Geometry: final body of the model. Coordinates: model frame, mm. Give positions to 0.01 mm unless a question says otherwise; leave off trailing zeros. Order: outer loops, then holes, each group sorted by start corner. A loop starts at its lowest first (then second) coordinate and runs counter-clockwise, first axis right, second up. Notation, with made-up numbers: (-29.5, 81.25) -> (12.5, 81.25) arc R29 cw to (12.5, 120.25) -> close; hole circle Ø11 at (86, 36.5). An arc over 180 degrees is marked (long way). One line per question, with ' | ' between items.
from build123d import *

# Parameters (mm, degrees)
ESQUISSE1_W             = 94.57
ESQUISSE1_H             = 60.88
BOSS_EXTRU_1_DEPTH      = 3.7
ESQUISSE2_W             = 88.629386258
ESQUISSE2_H             = 58.041323691
ENL_V_MAT_EXTRU_1_DEPTH = 0.05
ESQUISSE3_W             = 3.887425577
ESQUISSE3_H             = 19.495847756
BOSS_EXTRU_2_DEPTH      = 0.05
ESQUISSE4_W             = 3.887425577
ESQUISSE4_H             = 19.495847756
BOSS_EXTRU_3_DEPTH      = 0.1


with BuildPart() as part:
    # Esquisse1 → Boss.-Extru.1 (new body)
    with BuildSketch(Plane.XY):
        with Locations((47.285, 30.44)):
            Rectangle(ESQUISSE1_W, ESQUISSE1_H)
    extrude(amount=BOSS_EXTRU_1_DEPTH)

    # Esquisse2 → Enlèv. mat.-Extru.1 (cut)
    with BuildSketch(Plane.XY.offset(3.7)):
        with Locations((48.709909747, 30.392503009)):
            Rectangle(ESQUISSE2_W, ESQUISSE2_H)
    extrude(amount=-ENL_V_MAT_EXTRU_1_DEPTH, mode=Mode.SUBTRACT)

    # Esquisse3 → Boss.-Extru.2 (add)
    with BuildSketch(Plane(origin=(0, 0, 0), x_dir=(-1, 0, 0), z_dir=(0, 0, -1))):
        with BuildLine():
            Line((-9.099589702, 9.441066071), (0, 9.441066071))
            Line((0, 9.441066071), (0, 51.438933929))
            Line((0, 51.438933929), (-9.099589702, 51.438933929))
            ThreePointArc((-9.099589702, 51.438933929), (-10.513803264, 50.853147491), (-11.099589702, 49.438933929))
            Line((-11.099589702, 49.438933929), (-11.099589702, 42.94))
            ThreePointArc((-11.099589702, 42.94), (-11.68537614, 41.525786438), (-13.099589702, 40.94))
            Line((-13.099589702, 40.94), (-40, 40.94))
            Line((-40, 40.94), (-40, 19.94))
            Line((-40, 19.94), (-13.099589702, 19.94))
            ThreePointArc((-13.099589702, 19.94), (-11.68537614, 19.354213562), (-11.099589702, 17.94))
            Line((-11.099589702, 17.94), (-11.099589702, 11.441066071))
            ThreePointArc((-11.099589702, 11.441066071), (-10.513803264, 10.026852509), (-9.099589702, 9.441066071))
        make_face()
        with Locations((-37.941401464, 30.44)):
            Rectangle(ESQUISSE3_W, ESQUISSE3_H, mode=Mode.SUBTRACT)
    extrude(amount=BOSS_EXTRU_2_DEPTH)

    # Esquisse4 → Boss.-Extru.3 (add)
    with BuildSketch(Plane(origin=(0, 0, 0), x_dir=(-1, 0, 0), z_dir=(0, 0, -1))):
        with Locations((-37.941401464, 30.44)):
            Rectangle(ESQUISSE4_W, ESQUISSE4_H)
    extrude(amount=BOSS_EXTRU_3_DEPTH)


solid = part.part
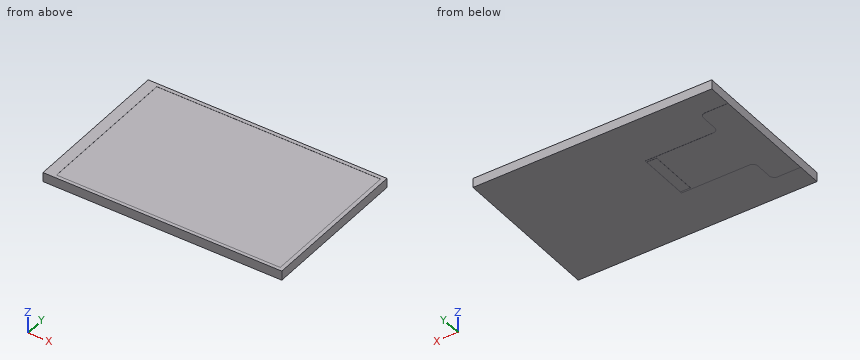
1) Section B-B on x = 65. Return loops of the section in (y, z).
Check result:
outline: (0, 0) -> (60.88, 0) -> (60.88, 3.7) -> (59.41, 3.7) -> (59.41, 3.65) -> (1.37, 3.65) -> (1.37, 3.7) -> (0, 3.7) -> close
2) Material intervals for probe 1 along Z at (x, y) = (18, 50.5), sorted ascending. Write a range as from..to.
Check result:
probe 1: z = 0..3.65
3) Section A-A on y = 12.5. Return loops of the section in (x, z).
Check result:
outline: (0, -0.05) -> (11.1, -0.05) -> (11.1, 0) -> (94.57, 0) -> (94.57, 3.7) -> (93.02, 3.7) -> (93.02, 3.65) -> (4.4, 3.65) -> (4.4, 3.7) -> (0, 3.7) -> close
4) Section C-C on y = 55. Return loops of the section in (x, z).
Check result:
outline: (0, 0) -> (94.57, 0) -> (94.57, 3.7) -> (93.02, 3.7) -> (93.02, 3.65) -> (4.4, 3.65) -> (4.4, 3.7) -> (0, 3.7) -> close
5) Contact query for flat-ended pins moving along their axis: pin 1 Ø1 at (y, z) = (7.5, 1) entering from -X; pin 2 Ø1.5 at (x, y) = (18, 11) entering from -Z; pin 3 Ø12 at (x, y) = (17.5, 20.5) entering from -Z; pin 4 Ø2 at (x, y) = (21, 45) entering from +Z. Output: stop coordinate, or through.
Check result:
pin 1: stops at x = 0 | pin 2: stops at z = 0 | pin 3: stops at z = -0.05 | pin 4: stops at z = 3.65
6) Section D-D on x = 15. Return loops of the section in (y, z).
Check result:
outline: (0, 0) -> (19.94, 0) -> (19.94, -0.05) -> (40.94, -0.05) -> (40.94, 0) -> (60.88, 0) -> (60.88, 3.7) -> (59.41, 3.7) -> (59.41, 3.65) -> (1.37, 3.65) -> (1.37, 3.7) -> (0, 3.7) -> close
